Work out the finished part from the listing and answer in its coordinate system (mm). A direction names the side the tool comes from. Round coordinates to 2 decimals unless told otherwise and drop trailing zeros. Loops run counter-clockwise (first coordinate to the right, second up) from the corner with the lowest first, then second, coordinate; pieces in that order, holes last.
```python
from build123d import *

# Parameters (mm, degrees)
F2_R     = 32
F2_R_2   = 12
F3_DEPTH = 5
F4_R     = 5
F5_DEPTH = 5


with BuildPart() as f1:
    # F0 (on Front) → F1 (revolve)
    with BuildSketch(Plane.XZ):
        Polygon((-50, 0), (-50, 434), (-10, 467.5639852471), (-10, 507.5639852471), (-12, 507.5639852471), (-12, 468.4966005634), (-52, 434.9326153163), (-52, -2), (0, -2), (0, 0), align=None)
    revolve(axis=Axis((0, 0, 216.0225092206), (0, 0, 1)))

    # F2 (on face) → F3 (join)
    with BuildSketch(Plane.XY.offset(507.5639852471)):
        Circle(F2_R)
        Circle(F2_R_2, mode=Mode.SUBTRACT)
    extrude(amount=-F3_DEPTH)

    # F4 (on face) → F5 (cut, through all)
    with BuildSketch(Plane.XY.offset(507.5639852471)):
        with Locations((0, 20)):
            Circle(F4_R)
        with Locations((-20, 0)):
            Circle(F4_R)
        with Locations((0, -20)):
            Circle(F4_R)
        with Locations((20, 0)):
            Circle(F4_R)
    extrude(amount=-F5_DEPTH, mode=Mode.SUBTRACT)


solid = f1.part
```
1. Find section A-A (y = 0). Write down the section's boundary in (x, z), then the cut area to 3 significant figures.
Answer key:
outline: (-52, -2) - (52, -2) - (52, 434.93) - (12, 468.5) - (12, 502.56) - (15, 502.56) - (15, 507.56) - (10, 507.56) - (10, 467.56) - (50, 434) - (50, 0) - (-50, 0) - (-50, 434) - (-10, 467.56) - (-10, 507.56) - (-15, 507.56) - (-15, 502.56) - (-12, 502.56) - (-12, 468.5) - (-52, 434.93) - close; (-32, 502.56) - (-25, 502.56) - (-25, 507.56) - (-32, 507.56) - close; (25, 502.56) - (32, 502.56) - (32, 507.56) - (25, 507.56) - close
area: 2,410 mm2
2. Determine the mould class of faces 4 (the face through (2.6, 11.7, 465.9)), 5 (the face through (7, 8, 507.564)), 6 (the face through (-6.94, -31.24, 505.1)) for opening direction Y: +Y half, -Y half, draft (parallel to the pull), parting line (faces both ways), or undercut.
Answer key:
face 4: undercut
face 5: draft
face 6: parting line
3. Consider probe 1 along Y at (x, z) = (0, 504.9); probe 2 along Z at (x, y) = (10.5, 15); probe 3 along Y at (x, z) = (-20, 506.5). Determine where each line is inside the solid, lowest interval first.
Answer key:
probe 1: y = -32 to -25, -15 to -10, 10 to 15, 25 to 32
probe 2: z = -2 to 0, 460.59 to 463.2, 502.56 to 507.56
probe 3: y = -24.98 to -5, 5 to 24.98
4. Find section C-C (x = -20). Give the number of separate pieces and of enclosed holes in the cut face, then the cut area to 3 significant figures.
Answer key:
separate pieces: 3
enclosed holes: 1
area: 2,530 mm2
5. Given pin 1 (1.5 mm diameter, centred on x = 22, y = 2, fed in from +Z); pin 2 (9 mm diameter, centred on x = 0, y = 20, fed in from +Z); pin 3 (8 mm diameter, centred on x = 20, y = 0, fed in from +Z), each flat-ended and moving along its own axis, determine where each tip first touches the part or whether it passes through.
Answer key:
pin 1: stops at z = 460.66
pin 2: stops at z = 465.56
pin 3: stops at z = 465.14
6. Which of the six approach directions +Z, -Z, +X, -X, +Y, -Y give full straight-line access (tool end or side, diameter ignored) to faces 1 (the face through (41.265, 31.641, 213.408)), 2 (the face through (10.689, -9.801, 466.397)), 3 (the face through (-1.08, -24.88, 505.1))?
Answer key:
face 1: +Z, -Z
face 2: none
face 3: +Z
7. Find section B-B (z = 338.5). Write down the section's boundary in (x, y).
Answer key:
outline: circle Ø104 at (0, 0); hole circle Ø100 at (0, 0)
